```python
from build123d import *

# Parameters (mm, degrees)
SKETCH_W  = 60
SKETCH_H  = 60
SKETCH_R  = 21
PAD_DEPTH = 1


with BuildPart() as pad:
    # Sketch → Pad (new body)
    with BuildSketch(Plane.XY):
        Rectangle(SKETCH_W, SKETCH_H)
        Circle(SKETCH_R, mode=Mode.SUBTRACT)
    extrude(amount=PAD_DEPTH)


with BuildPart() as cone:
    # Cone → Cone (revolve)
    with BuildSketch(Plane.XZ):
        Polygon((0, 0), (20, 0), (27, 15), (0, 15), align=None)
    revolve(axis=Axis((0, 0, 0), (0, 0, 1)))


with BuildPart() as fusion:
    # Cone001 → Cone001 (revolve)
    with BuildSketch(Plane.XZ):
        Polygon((0, 0), (21, 0), (28, 15), (0, 15), align=None)
    revolve(axis=Axis((0, 0, 0), (0, 0, 1)))

    # Cut: cut Cone
    add(cone.part, mode=Mode.SUBTRACT)

    # Fusion: union Pad
    add(pad.part)


solid = fusion.part
```
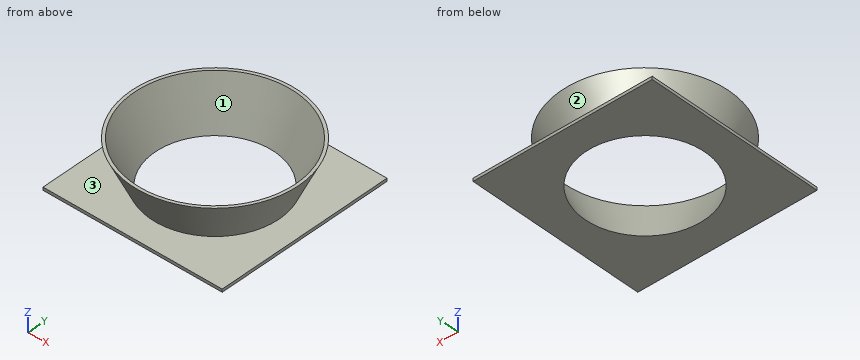
Source: CAD feature listing. Evaluate the final solid. Frame: model axes, mm. Face numbers are marked on the shaded views. Coordinates: 2 decimals unless noted, no trailing zeros. Write each loop counter-clockwise with the first axis right and the second up, starting at its lowest first coordinate (ties: lowest second). Pieces come first, ordered by that corner, then holes. Notation, with made-up numbers: M 89.5,-5.75 L 135.5,-5.75 A37 ccw 135.5,31.25 Z; hole C 32,25.25 d11. An arc over 180 degrees is marked long. Answer as a JSON object with one key per item and string values.
1. Draft query along Y for the marked faces 1, 2 and 3. Return one class per face: released by +Y, released by -Y, zero draft, split by the parting line, or undercut.
Evaluation:
{"face 1": "undercut", "face 2": "split by the parting line", "face 3": "zero draft"}
2. Cut plane B-B on z = 5.25. Output: boundary loops of the cut face in (x, y).
Evaluation:
{"outline": "C 0,0 d46.9; hole C 0,0 d44.9"}
3. Cut plane A-A on y = 0. Output: boundary loops of the cut face in (x, z), plus the area to 3 significant figures.
Evaluation:
{"outline": "M -30,0 L -20,0 L -27,15 L -28,15 L -21.47,1 L -30,1 Z; M 20,0 L 30,0 L 30,1 L 21.47,1 L 28,15 L 27,15 Z", "area": "47.5 mm^2"}
4. Cut plane D-D on z = 9.25. Output: boundary loops of the cut face in (x, y).
Evaluation:
{"outline": "C 0,0 d50.63; hole C 0,0 d48.63"}
5. Ray query, L1, parallel to Y at x = 5, z = 4.75; L2, parallel to Z at x = 23, y = -4; L3, parallel to X at y = -6.5, z = 3.75. Return the intervals inside material, ascending.
Evaluation:
{"L1": "-22.67 to -21.65, 21.65 to 22.67", "L2": "0 to 1, 5.03 to 7.17", "L3": "-21.8 to -20.76, 20.76 to 21.8"}
6. Contact query for flat-ended pins moving along their axis: P1, Ø1, axis at y = -4, z = 7, coming from the -X side; P2, Ø2, axis at y = -5.5, z = 13, coming from the -X side; P3, Ø1, axis at y = -20.5, z = 3, coming from the -X side. Output: stop coordinate, or through.
Evaluation:
{"P1": "x = -24.18", "P2": "x = -27.02", "P3": "x = -10.21"}
